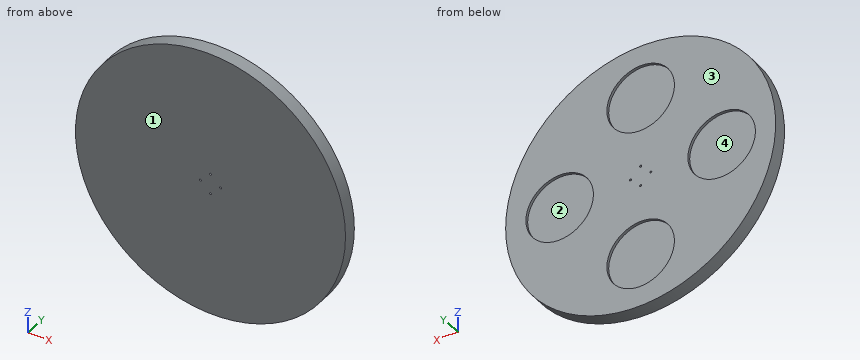
from build123d import *

# Parameters (mm, degrees)
CROQUIS1_R              = 100
SALIENTE_EXTRUIR1_DEPTH = 10
CROQUIS2_R              = 0.75
CORTAR_EXTRUIR1_DEPTH   = 11
CROQUIS3_R              = 25
CORTAR_EXTRUIR2_DEPTH   = 2


with BuildPart() as part:
    # Croquis1 → Saliente-Extruir1 (new body)
    with BuildSketch(Plane(origin=(0, 0, 0), x_dir=(1, 0, 0), z_dir=(0, 1, 0))):
        Circle(CROQUIS1_R)
    extrude(amount=SALIENTE_EXTRUIR1_DEPTH)

    # Croquis2 → Cortar-Extruir1 (cut, through all)
    with BuildSketch(Plane(origin=(0, 10, 0), x_dir=(1, 0, 0), z_dir=(0, 1, 0))):
        with Locations((-7.5, 0)):
            Circle(CROQUIS2_R)
        with Locations((0, -7.5)):
            Circle(CROQUIS2_R)
        with Locations((7.5, 0)):
            Circle(CROQUIS2_R)
        with Locations((0, 7.5)):
            Circle(CROQUIS2_R)
    extrude(amount=-CORTAR_EXTRUIR1_DEPTH, mode=Mode.SUBTRACT)

    # Croquis3 → Cortar-Extruir2 (cut)
    with BuildSketch(Plane(origin=(0, 10, 0), x_dir=(1, 0, 0), z_dir=(0, 1, 0))):
        with Locations((-60, 0)):
            Circle(CROQUIS3_R)
        with Locations((0, 60)):
            Circle(CROQUIS3_R)
        with Locations((60, 0)):
            Circle(CROQUIS3_R)
        with Locations((0, -60)):
            Circle(CROQUIS3_R)
    extrude(amount=-CORTAR_EXTRUIR2_DEPTH, mode=Mode.SUBTRACT)


solid = part.part
Can you work these out from the model? Positions are in its coordinate system, mm. Face numbers are marked on the shaded views. A direction names the side the tool comes from. Coordinates: 2 decimals unless noted, no trailing zeros. Write each loop counter-clockwise with the first axis right and the second up, starting at its lowest first coordinate (ties: lowest second). Pieces come first, ordered by that corner, then holes.
Q1. Which directions (+Z, -Z, +X, -X, +Y, -Y) give clear straight access to the entire face, cutting with the end or side of a thin tool? Please do the marked faces 3 and 4.
Results found:
face 3: +Z, -Z, +X, -X, +Y
face 4: +Y
Q2. If we mould it in two halves opening along Z, with no side actions, what happens to the marked faces 1 and 2? For each: +Z half, -Z half, draft (parallel to the pull), parting line (faces both ways), or undercut.
Results found:
face 1: draft
face 2: undercut
Q3. Imagine slicing it at A-A, the plane z = 60. List the corners of the cut face in (x, y) for me, plus the area to 3 significant figures.
Results found:
outline: (-80, 0) - (80, 0) - (80, 10) - (25, 10) - (25, 8) - (-25, 8) - (-25, 10) - (-80, 10) - close
area: 1,500 mm2
Q4. Imagine slicing it at B-B, the plane x = -60. List the corners of the cut face in (y, z) for me.
Results found:
outline: (0, -80) - (10, -80) - (10, -25) - (8, -25) - (8, 25) - (10, 25) - (10, 80) - (0, 80) - close
Q5. Imagine slicing it at C-C, the plane y = 3.5. List the corners of the cut face in (x, z) for me.
Results found:
outline: circle Ø200 at (0, 0); hole circle Ø1.5 at (-7.5, 0); hole circle Ø1.5 at (0, -7.5); hole circle Ø1.5 at (0, 7.5); hole circle Ø1.5 at (7.5, 0)
Q6. For P1, Ø1, axis at y = 7, z = 74.5, coming from the +X side; P2, Ø15, axis at x = -67, z = -5, coming from the +Y side; P3, Ø5, axis at x = 8, y = 5, coming from the +Z side, each with a flat end and sliding along its axis, tell me the tip position at first contact or that it passes through.
Results found:
P1: stops at x = 67.26
P2: stops at y = 8
P3: stops at z = 99.85
Q7. Imagine slicing it at D-D, the plane z = -13. List the corners of the cut face in (x, y) for me.
Results found:
outline: (-99.15, 0) - (99.15, 0) - (99.15, 10) - (81.35, 10) - (81.35, 8) - (38.65, 8) - (38.65, 10) - (-38.65, 10) - (-38.65, 8) - (-81.35, 8) - (-81.35, 10) - (-99.15, 10) - close
Q8. Please list where these lines run through material, in increasing order: L1, parallel to Z at x = 0, y = 3.5; L2, parallel to Z at x = -7.5, y = 5.75; L3, parallel to Z at x = 60, y = 9.3.
Results found:
L1: z = -100 to -8.25, -6.75 to 6.75, 8.25 to 100
L2: z = -99.72 to -0.75, 0.75 to 99.72
L3: z = -80 to -25, 25 to 80
